Part print with two shaded views. Sizes in mm from the minimum x, y, z corner. A direction names the side the tool comes from. Round coordinates to 2 decimals unless told otherwise and drop trailing zeros. Order: outer loops, then holes, each group sorted by start corner. A loop starts at its lowest first (then second) coordinate and runs counter-clockwise, first axis right, second up. Notation, with made-up numbers: M 52,-3.5 L 85,-3.5 A26 ccw 85,32.5 Z; hole C -39,28 d5. An arc over 180 degrees is marked long. One line per question, with ' | ' between items. Start each with the question number.
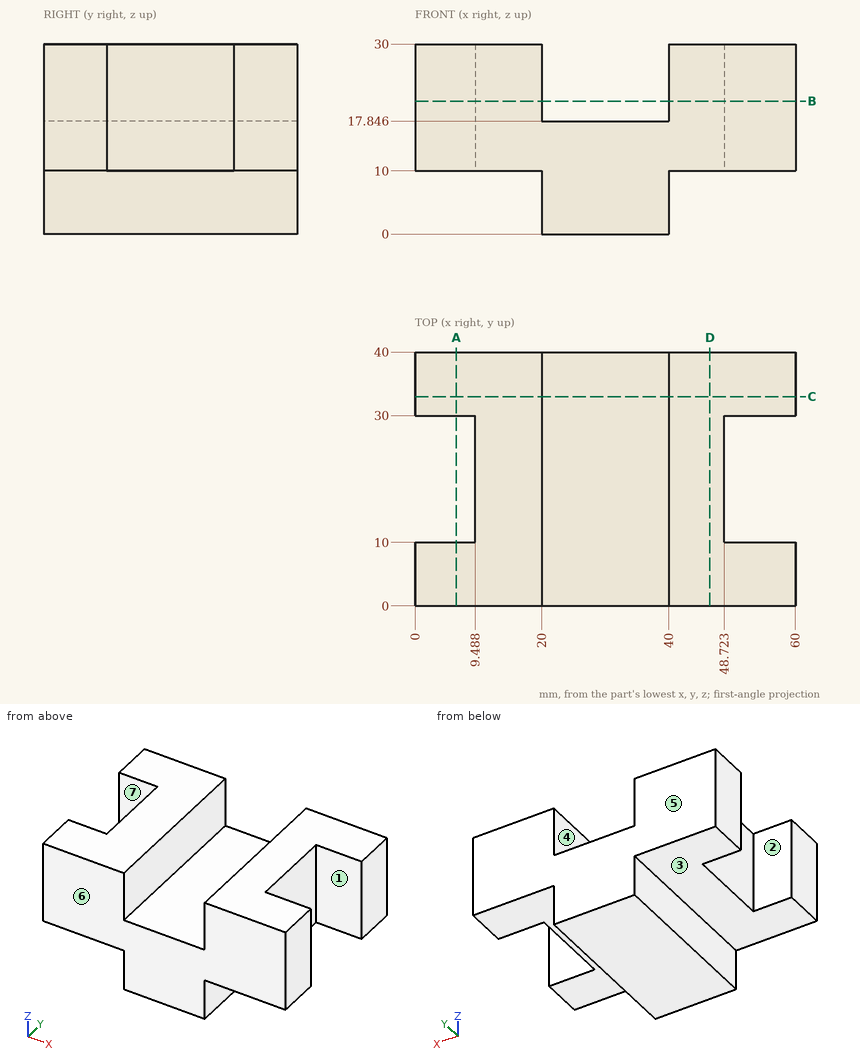
Item 1: Cut at C-C on y = 33. Write the cut outline in (x, z).
Item 2: Cut at A-A on x = 6.5. Write the cut outline in (y, z), then the cut area to 3 significant figures.
Item 3: Cut at B-B on z = 21. Write the cut outline in (x, y), then the cut area to 3 significant figures.
Item 4: Flat gauge pins, fed straight in: pin 1 (16 mm diameter, centred on y = 21, z = 20.5, fed in from -X); pin 2 (3 mm diameter, centred on y = 28.5, z = 5.5, fed in from -X); pin 3 (10 mm diameter, centred on x = 12, y = 14.5, fed in from -Z). Where does each tip first touch, or does it go through?
Item 5: Wall check: line 1 along Y through (x, z) = (52, 19); line 2 along X through (y, z) = (28, 23); line 3 along X through (y, z) = (4, 19). Give the ranges that are in metal, low to high. Write a range as [from, to].
Item 6: Cut at D-D on x = 46.5. Write the cut outline in (y, z).
Item 7: Tool access for the marked faces 1, 2, 3 and 4: list every direction of +Z, -Z, +X, -X, +Y, -Y with a clear straight run to the whole face (end or side of a thin tool).
Item 8: Two-plate mould, pull along Y, no slides. Class the marked faces 5, 6 and 7: +Y half, -Y half, draft (parallel to the pull), parting line (faces both ways), or undercut.
Results found:
1) outline: M 0,10 L 20,10 L 20,0 L 40,0 L 40,10 L 60,10 L 60,30 L 40,30 L 40,17.85 L 20,17.85 L 20,30 L 0,30 Z
2) outline: M 0,10 L 10,10 L 10,30 L 0,30 Z; M 30,10 L 40,10 L 40,30 L 30,30 Z | area: 400 mm^2
3) outline: M 0,0 L 20,0 L 20,40 L 0,40 L 0,30 L 9.49,30 L 9.49,10 L 0,10 Z; M 40,0 L 60,0 L 60,10 L 48.72,10 L 48.72,30 L 60,30 L 60,40 L 40,40 Z | area: 1,180 mm^2
4) pin 1: stops at x = 9.49 | pin 2: stops at x = 20 | pin 3: stops at z = 10
5) line 1: y = [0, 10], [30, 40] | line 2: x = [9.49, 20], [40, 48.72] | line 3: x = [0, 20], [40, 60]
6) outline: M 0,10 L 40,10 L 40,30 L 0,30 Z
7) face 1: +Z, -Z, +X | face 2: +Z, -Z, -X | face 3: -Z, -X, +Y, -Y | face 4: +Z, +Y, -Y
8) face 5: +Y half | face 6: -Y half | face 7: undercut
